```python
from build123d import *

# Parameters (mm, degrees)
SKETCH1_R              = 1.5
BOSS_EXTRUDE1_DEPTH    = 2
BOSS_EXTRUDE1_2_DEPTH  = 2
BOSS_EXTRUDE1_3_DEPTH  = 2
BOSS_EXTRUDE1_4_DEPTH  = 2
BOSS_EXTRUDE1_5_DEPTH  = 2
BOSS_EXTRUDE1_6_DEPTH  = 2
BOSS_EXTRUDE1_7_DEPTH  = 2
BOSS_EXTRUDE1_8_DEPTH  = 2
BOSS_EXTRUDE1_9_DEPTH  = 2
BOSS_EXTRUDE1_10_DEPTH = 2
BOSS_EXTRUDE1_11_DEPTH = 2
BOSS_EXTRUDE1_12_DEPTH = 2
SKETCH1_3_W            = 30
SKETCH1_3_H            = 10
BOSS_EXTRUDE2_DEPTH    = 1
SKETCH1_4_W            = 30
SKETCH1_4_H            = 10
SKETCH1_4_W_2          = 28
SKETCH1_4_H_2          = 8
SKETCH1_4_R            = 2.035533906
SKETCH1_4_R_2          = 1.5
BOSS_EXTRUDE3_DEPTH    = 1


with BuildPart() as part:
    # Sketch1 → Boss-Extrude1 (new body)
    with BuildSketch(Plane(origin=(0, 0, 0), x_dir=(1, 0, 0), z_dir=(0, 1, 0))):
        with Locations((-2.5, 2.5)):
            Circle(SKETCH1_R)
    extrude(amount=BOSS_EXTRUDE1_DEPTH)



with BuildPart() as body_2:
    # Sketch1 → Boss-Extrude1 2 (new body)
    with BuildSketch(Plane(origin=(0, 0, 0), x_dir=(1, 0, 0), z_dir=(0, 1, 0))):
        with Locations((-7.5, 2.5)):
            Circle(SKETCH1_R)
    extrude(amount=BOSS_EXTRUDE1_2_DEPTH)


with BuildPart() as body_3:
    # Sketch1 → Boss-Extrude1 3 (new body)
    with BuildSketch(Plane(origin=(0, 0, 0), x_dir=(1, 0, 0), z_dir=(0, 1, 0))):
        with Locations((-12.5, 2.5)):
            Circle(SKETCH1_R)
    extrude(amount=BOSS_EXTRUDE1_3_DEPTH)


with BuildPart() as body_4:
    # Sketch1 → Boss-Extrude1 4 (new body)
    with BuildSketch(Plane(origin=(0, 0, 0), x_dir=(1, 0, 0), z_dir=(0, 1, 0))):
        with Locations((-12.5, -2.5)):
            Circle(SKETCH1_R)
    extrude(amount=BOSS_EXTRUDE1_4_DEPTH)


with BuildPart() as body_5:
    # Sketch1 → Boss-Extrude1 5 (new body)
    with BuildSketch(Plane(origin=(0, 0, 0), x_dir=(1, 0, 0), z_dir=(0, 1, 0))):
        with Locations((-7.5, -2.5)):
            Circle(SKETCH1_R)
    extrude(amount=BOSS_EXTRUDE1_5_DEPTH)


with BuildPart() as body_6:
    # Sketch1 → Boss-Extrude1 6 (new body)
    with BuildSketch(Plane(origin=(0, 0, 0), x_dir=(1, 0, 0), z_dir=(0, 1, 0))):
        with Locations((-2.5, -2.5)):
            Circle(SKETCH1_R)
    extrude(amount=BOSS_EXTRUDE1_6_DEPTH)


with BuildPart() as body_7:
    # Sketch1 → Boss-Extrude1 7 (new body)
    with BuildSketch(Plane(origin=(0, 0, 0), x_dir=(1, 0, 0), z_dir=(0, 1, 0))):
        with Locations((2.5, 2.5)):
            Circle(SKETCH1_R)
    extrude(amount=BOSS_EXTRUDE1_7_DEPTH)


with BuildPart() as body_8:
    # Sketch1 → Boss-Extrude1 8 (new body)
    with BuildSketch(Plane(origin=(0, 0, 0), x_dir=(1, 0, 0), z_dir=(0, 1, 0))):
        with Locations((7.5, 2.5)):
            Circle(SKETCH1_R)
    extrude(amount=BOSS_EXTRUDE1_8_DEPTH)


with BuildPart() as body_9:
    # Sketch1 → Boss-Extrude1 9 (new body)
    with BuildSketch(Plane(origin=(0, 0, 0), x_dir=(1, 0, 0), z_dir=(0, 1, 0))):
        with Locations((12.5, 2.5)):
            Circle(SKETCH1_R)
    extrude(amount=BOSS_EXTRUDE1_9_DEPTH)


with BuildPart() as body_10:
    # Sketch1 → Boss-Extrude1 10 (new body)
    with BuildSketch(Plane(origin=(0, 0, 0), x_dir=(1, 0, 0), z_dir=(0, 1, 0))):
        with Locations((12.5, -2.5)):
            Circle(SKETCH1_R)
    extrude(amount=BOSS_EXTRUDE1_10_DEPTH)


with BuildPart() as body_11:
    # Sketch1 → Boss-Extrude1 11 (new body)
    with BuildSketch(Plane(origin=(0, 0, 0), x_dir=(1, 0, 0), z_dir=(0, 1, 0))):
        with Locations((7.5, -2.5)):
            Circle(SKETCH1_R)
    extrude(amount=BOSS_EXTRUDE1_11_DEPTH)


with BuildPart() as body_12:
    # Sketch1 → Boss-Extrude1 12 (new body)
    with BuildSketch(Plane(origin=(0, 0, 0), x_dir=(1, 0, 0), z_dir=(0, 1, 0))):
        with Locations((2.5, -2.5)):
            Circle(SKETCH1_R)
    extrude(amount=BOSS_EXTRUDE1_12_DEPTH)


with BuildPart() as part_1:
    add(part.part)

    add(body_2.part)  # Boss-Extrude2 merges body 2

    add(body_3.part)  # Boss-Extrude2 merges body 3

    add(body_4.part)  # Boss-Extrude2 merges body 4

    add(body_5.part)  # Boss-Extrude2 merges body 5

    add(body_6.part)  # Boss-Extrude2 merges body 6

    add(body_7.part)  # Boss-Extrude2 merges body 7

    add(body_8.part)  # Boss-Extrude2 merges body 8

    add(body_9.part)  # Boss-Extrude2 merges body 9

    add(body_10.part)  # Boss-Extrude2 merges body 10

    add(body_11.part)  # Boss-Extrude2 merges body 11

    add(body_12.part)  # Boss-Extrude2 merges body 12
    # Sketch1_3 → Boss-Extrude2 (add)
    with BuildSketch(Plane(origin=(0, 0, 0), x_dir=(1, 0, 0), z_dir=(0, 1, 0))):
        Rectangle(SKETCH1_3_W, SKETCH1_3_H)
    extrude(amount=BOSS_EXTRUDE2_DEPTH)

    # Sketch1_4 → Boss-Extrude3 (add)
    with BuildSketch(Plane(origin=(0, 0, 0), x_dir=(1, 0, 0), z_dir=(0, 1, 0))):
        Rectangle(SKETCH1_4_W, SKETCH1_4_H)
        Rectangle(SKETCH1_4_W_2, SKETCH1_4_H_2, mode=Mode.SUBTRACT)
        with Locations((-10, 0)):
            Circle(SKETCH1_4_R)
        with Locations((-10, 0)):
            Circle(SKETCH1_4_R_2, mode=Mode.SUBTRACT)
        with Locations((-5, 0)):
            Circle(SKETCH1_4_R)
        with Locations((-5, 0)):
            Circle(SKETCH1_4_R_2, mode=Mode.SUBTRACT)
        Circle(SKETCH1_4_R)
        Circle(SKETCH1_4_R_2, mode=Mode.SUBTRACT)
        with Locations((5, 0)):
            Circle(SKETCH1_4_R)
        with Locations((5, 0)):
            Circle(SKETCH1_4_R_2, mode=Mode.SUBTRACT)
        with Locations((10, 0)):
            Circle(SKETCH1_4_R)
        with Locations((10, 0)):
            Circle(SKETCH1_4_R_2, mode=Mode.SUBTRACT)
    extrude(amount=-BOSS_EXTRUDE3_DEPTH)


solid = part_1.part
```
Could you check a few things on this model? Use its own coordinates, in mm. A direction names the side the tool comes from. Round coordinates to 2 decimals unless told otherwise and drop trailing zeros. Write each loop counter-clockwise with the first axis right and the second up, starting at its lowest first coordinate (ties: lowest second). Pieces come first, ordered by that corner, then holes. Notation, with made-up numbers: M 1,-18.5 L 30,-18.5 A33 ccw 30,18.5 Z; hole C 15,37 d10. An arc over 180 degrees is marked long. Answer in a Markdown table with one row per item. Add a question column.
Q1. Will these pins go through, and if not, where does the flat tip stop? pin 1 Ø1.5 at (x, z) = (5.5, 0.5) entering from -Y; pin 2 Ø5 at (x, z) = (-10, 0) entering from -Y; pin 3 Ø4 at (x, z) = (10, 0) entering from +Y.
Q2. Imagine slicing it at D-D (x = 12.5). Please give me the cut outline in (y, z).
Q3. On a 3-axis mill with a long thin cutter (end or side, diameter ignored), from which of +Z, -Z, +X, -X, +Y, -Y can I reach the whole of each face in a straight line? I mean faces 1 (the flat face through (-5, 0, 0)), 2 (the cylindrical face through (6.3, 1.5, -1.6)), 3 (the flat face through (-15, 0, 0)). Say none if no direction works.
Q4. If we mould it in two halves opening along Z, with no side actions, what happens to faces 4 (the flat face through (12, 2, 2)), 5 (the cylindrical face through (-6.2, -0.5, 0.9))? For each: +Z half, -Z half, draft (parallel to the pull), parting line (faces both ways), or undercut.
Q5. Imagine slicing it at A-A (x = -10). Please give me the cut outline in (y, z).
Q6. If I drill on line 1 (Z direction, x = 0, y = -0.5); line 2 (X direction, y = 1.8, z = -2.5); line 3 (Z direction, x = -0.5, y = -0.3), over which ranges is the centre line in solid material (lowest first)? Write a range as from..to.
Q7. Imagine slicing it at B-B (y = 1.3). Give the number of separate pieces and of enclosed holes in the cut face, then the cut area to 3 significant figures.
Values:
| question | item | result |
|---|---|---|
| 1 | pin 1 | y = 0 |
| 1 | pin 2 | y = -1 |
| 1 | pin 3 | y = 1 |
| 2 | outline | M -1,-5 L 1,-5 L 1,-4 L 2,-4 L 2,-1 L 1,-1 L 1,1 L 2,1 L 2,4 L 1,4 L 1,5 L -1,5 L -1,4 L 0,4 L 0,-4 L -1,-4 Z |
| 3 | face 1 | -Y |
| 3 | face 2 | +Y |
| 3 | face 3 | +Z, -Z, -X, +Y, -Y |
| 4 | face 4 | draft |
| 4 | face 5 | undercut |
| 5 | outline | M -1,-5 L 1,-5 L 1,5 L -1,5 L -1,4 L 0,4 L 0,2.04 L -1,2.04 L -1,1.5 L 0,1.5 L 0,-1.5 L -1,-1.5 L -1,-2.04 L 0,-2.04 L 0,-4 L -1,-4 Z |
| 6 | line 1 | -5..-4, -2.04..-1.5, 1.5..2.04, 4..5 |
| 6 | line 2 | -14..-11, -9..-6, -4..-1, 1..4, 6..9, 11..14 |
| 6 | line 3 | -5..-4, -1.97..-1.41, 1.41..1.97, 4..5 |
| 7 | separate pieces | 12 |
| 7 | enclosed holes | 0 |
| 7 | area | 84.8 mm^2 |
